Job drawing, mm, ordinate dimensions from the low corner. One solid piece. A direction names the side the tool comes from. Give positions to 0.01 mm unless a question says otherwise; leave off trailing zeros. Loops run counter-clockwise (first coordinate to the right, second up) from the corner with the lowest first, then second, coordinate; pieces in that order, holes last.
Item 1: Saw through at A-A on z = 7.5. Give the cut face in (x, y), plus the area to 3 significant figures.
Item 2: Saw through at C-C on x = 17. Give the cut face in (y, z), plus the area to 3 significant figures.
Item 3: Mould opens along Z. For the marked faces 1 and 2 say: released by +Z, released by -Z, zero draft, split by the parting line, or undercut.
Item 4: Drop flat-ended pins along their axis: P1, Ø19.5, axis at x = 7.5, z = 7.5, coming from the +Y side; P2, Ø2, axis at x = 73.5, y = 5.5, coming from the -Z side; P3, Ø6, axis at x = 70.5, z = 29, coming from the +Y side. Give the stop position or say it passes through.
Item 5: Which spindle directions (+Z, -Z, +X, -X, +Y, -Y) get a long thin tool onto all of the face, cutting with end or side? Do the marked faces 3 and 4. Say none if no direction does.
Item 6: Probe probe 1 along Z at (x, y) = (7.5, 3.85); probe 2 along Z at (x, y) = (7.5, 5.55); probe 3 along X at (y, z) = (3.95, 95.6). List the from-to ranges inside material, lowest first.
Item 7: Saw through at D-D on z = 92. Give the cut face in (x, y).
Item 8: Saw through at B-B on x = 7.5. Give the number of separate pieces and of enclosed holes in the cut face, plus the area to 3 significant figures.
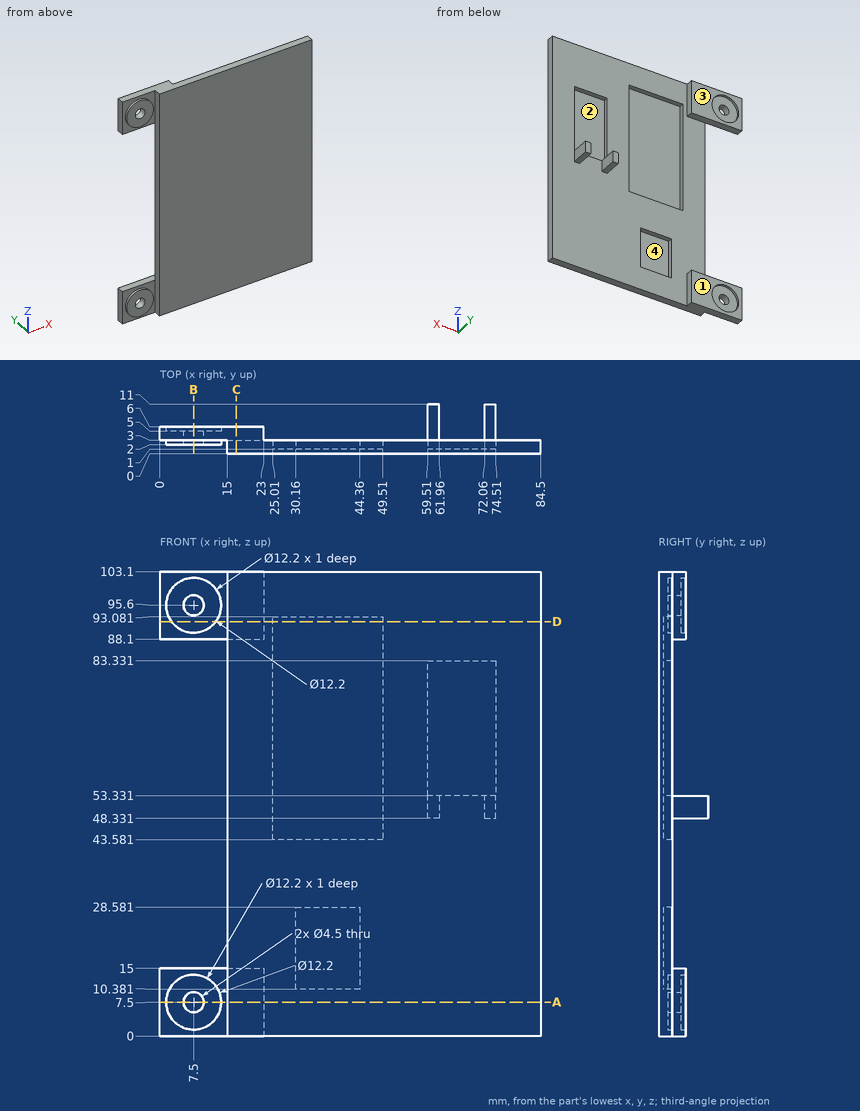
Results below:
1. outline: (0, 3) - (1.4, 3) - (1.4, 2) - (5.25, 2) - (5.25, 5) - (1.4, 5) - (1.4, 6) - (0, 6) - close; (9.75, 2) - (13.6, 2) - (13.6, 3) - (15, 3) - (15, 0) - (84.5, 0) - (84.5, 3) - (23, 3) - (23, 6) - (13.6, 6) - (13.6, 5) - (9.75, 5) - close
1. area: 264 mm2
2. outline: (0, 0) - (6, 0) - (6, 15) - (3, 15) - (3, 88.1) - (6, 88.1) - (6, 103.1) - (0, 103.1) - close
2. area: 399 mm2
3. face 1: zero draft
3. face 2: undercut
4. P1: stops at y = 6
4. P2: stops at z = 48.33
4. P3: stops at y = 3
5. face 3: +Z, -Z, +X, -X, +Y
5. face 4: +Y
6. probe 1: z = 0 to 5.25, 9.75 to 15, 88.1 to 93.35, 97.85 to 103.1
6. probe 2: z = 0 to 1.4, 13.6 to 15, 88.1 to 89.5, 101.7 to 103.1
6. probe 3: x = 0 to 5.25, 9.75 to 23
7. outline: (0, 3) - (2.58, 3) - (2.58, 2) - (12.42, 2) - (12.42, 3) - (15, 3) - (15, 0) - (84.5, 0) - (84.5, 3) - (49.51, 3) - (49.51, 1) - (25.01, 1) - (25.01, 3) - (23, 3) - (23, 6) - (12.42, 6) - (12.42, 5) - (2.58, 5) - (2.58, 6) - (0, 6) - close
8. separate pieces: 4
8. enclosed holes: 0
8. area: 63.0 mm2
